Study the drawing (mm; zero at the part's minimum x, y, z) and answer. A direction names the side the tool comes from. Give positions to 0.01 mm unless a question says otherwise; leave off trailing zeros. Write each loop counter-clockwise with the first axis right and the second up, starting at its lowest first coordinate (ties: lowest second). Pieces come first, ordered by that corner, then holes.
1) Given pin 1 Ø1.5 at (x, y) = (6, 4.5) entering from +Z; pin 2 Ø1.5 at (x, z) = (15, 7) entering from +Y; pin 3 Ø6 at (x, y) = (5, 5.5) entering from +Z; pin 4 Ø1.5 at (y, z) = (10, 4.5) entering from -X, each flat-ended and moving along its own axis, determine where each tip first touches the part or whether it passes through.
2) Straight lines are drawn through the part: probe 1 along Y at (x, z) = (25, 2.35); probe 2 along X at (y, z) = (2, 7.25); probe 3 along Z at (x, y) = (8, 3). For each, find the intervals that lie inside material, in ascending order.
3) A tool of negligible diameter and unlimited length cuts with its end or side. For the marked faces 4, 5, 6, 7 and 8, from which of +Z, -Z, +X, -X, +Y, -Y can it reach the whole face along a straight path? Write none if from no direction.
4) Find section C-C (x = 16.5). Determine the outline of the cut face in (y, z), plus the area to 3 significant figures.
5) Determine the mould class of the marked faces 1, 2 and 3 for opening direction X: pulls with the +X half, pulls with the -X half, needs draft (parallel to the pull), parting line crosses it, or undercut.
6) Find section A-A (x = 5). Determine the outline of the cut face in (y, z).
7) Find section D-D (y = 9.25). Determine the outline of the cut face in (x, z).
8) Find section B-B (y = 5.5). Determine the outline of the cut face in (x, z).
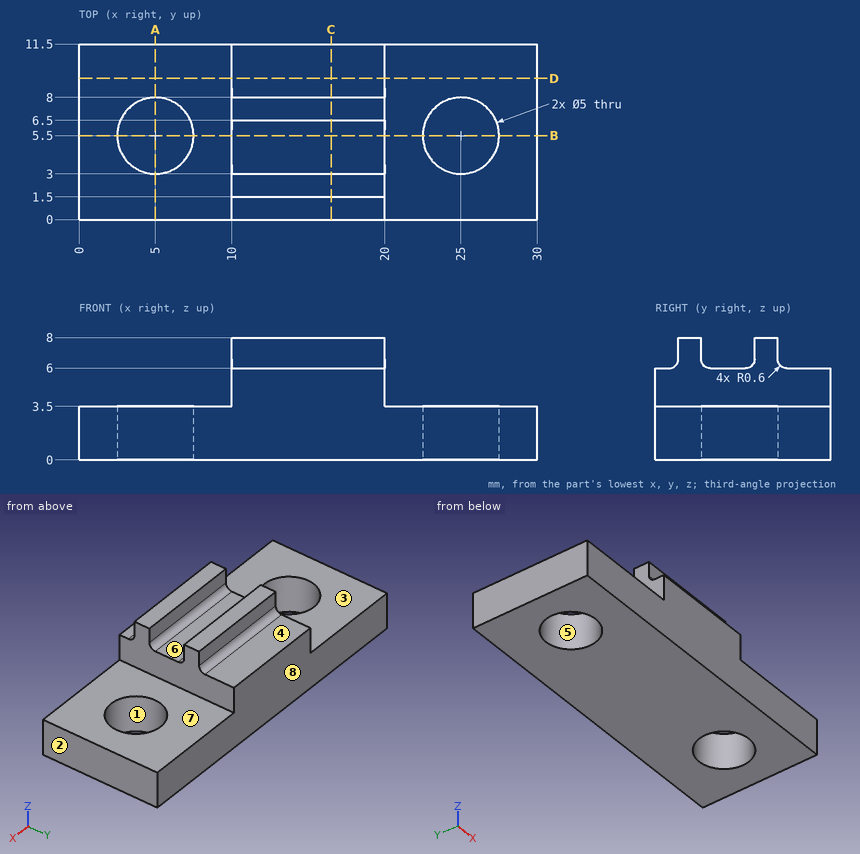
Results:
1. pin 1: passes through
1. pin 2: stops at y = 8.11
1. pin 3: stops at z = 3.5
1. pin 4: stops at x = 10
2. probe 1: y = 0 to 3, 8 to 11.5
2. probe 2: x = 10 to 20
2. probe 3: z = 0 to 3.5
3. face 4: +Z, +X, -X, +Y
3. face 5: +Z, -Z
3. face 6: +Z, +X, -X
3. face 7: +Z, +X, +Y, -Y
3. face 8: +Z, -Z, +X, -X, +Y
4. outline: (0, 0) - (11.5, 0) - (11.5, 6) - (8.6, 6) arc R0.6 cw to (8, 6.6) - (8, 8) - (6.5, 8) - (6.5, 6.6) arc R0.6 cw to (5.9, 6) - (3.6, 6) arc R0.6 cw to (3, 6.6) - (3, 8) - (1.5, 8) - (1.5, 6.6) arc R0.6 cw to (0.9, 6) - (0, 6) - close
4. area: 75.3 mm2
5. face 1: undercut
5. face 2: pulls with the +X half
5. face 3: needs draft
6. outline: (0, 0) - (3, 0) - (3, 3.5) - (0, 3.5) - close; (8, 0) - (11.5, 0) - (11.5, 3.5) - (8, 3.5) - close
7. outline: (0, 0) - (30, 0) - (30, 3.5) - (20, 3.5) - (20, 6) - (10, 6) - (10, 3.5) - (0, 3.5) - close
8. outline: (0, 0) - (2.5, 0) - (2.5, 3.5) - (0, 3.5) - close; (7.5, 0) - (22.5, 0) - (22.5, 3.5) - (20, 3.5) - (20, 6) - (10, 6) - (10, 3.5) - (7.5, 3.5) - close; (27.5, 0) - (30, 0) - (30, 3.5) - (27.5, 3.5) - close
